Could you check a few things on this model? Use its own coordinates, in mm. Face numbers are marked on the shaded views. Give positions to 0.01 mm unless a question says otherwise; leave off trailing zeros. Order: outer loops, then holes, each group sorted by start corner. A loop starts at its lowest first (then second) coordinate and runs counter-clockwise, first axis right, second up.
(1) Imagine slicing it at A-A, the plane x = -0.5. Write out the boundary of the cut face in (y, z), then the cut area to 3 significant figures.
(2) Will these pins go through, and if not, where does the flat tip stop? pin 1 (3 mm diameter, centred on x = 11.5, z = -28.5, fed in from +Y); pin 2 (0.6 mm diameter, centred on y = 1.5, z = -25.5, fed in from -X); pin 3 (2 mm diameter, centred on y = 9, z = -24, fed in from -X).
(3) Imagine slicing it at C-C, the plane z = -13. Write out the boundary of the cut face in (x, y).
(4) If we mould it in two halves opening along Y, with no side actions, what happens to the marked faces 1, 2 and 3? For each: released by +Y, released by -Y, zero draft, split by the parting line, or undercut.
(5) Imagine slicing it at B-B, the plane y = 7. Write out the boundary of the cut face in (x, z).
(6) If I drill on probe 1 along X at (y, z) = (1, -34); probe 2 along Z at (x, y) = (15, 7.25); probe 3 along Y at (x, z) = (5.25, -31), over which ranges is the centre line in solid material (lowest first)?
(7) Imagine slicing it at D-D, the plane x = 2.5. Write out the boundary of the cut face in (y, z), then the cut area to 3 significant figures.
from build123d import *

# Parameters (mm, degrees)
SKETCH1_R           = 1.75
BOSS_EXTRUDE1_DEPTH = 2
SKETCH4_W           = 2
SKETCH4_H           = 36.35059407
BOSS_EXTRUDE3_DEPTH = 10
CUT_EXTRUDE1_DEPTH  = 10
FILLET1_R           = 3


with BuildPart() as part:
    # Sketch1 → Boss-Extrude1 (new body)
    with BuildSketch(Plane(origin=(0, 0, 0), x_dir=(1, 0, 0), z_dir=(0, 1, 0))):
        Polygon((5.603006234, 2.519255437), (16.866529546, 2.519255437), (16.866529546, 38.869849507), (4.37040298, 38.869849507), (-1.929271174, 38.869849507), (-1.929271174, 30.775756588), (6.866529546, 30.775756588), (6.866529546, 19.460556696), (-1.929271174, 19.460556696), (-1.929271174, 2.519255437), align=None)
        with Locations(Location((2.868105939, 34.070567936, 0), (0, 0, 270))):
            Circle(SKETCH1_R, mode=Mode.SUBTRACT)
        with Locations(Location((2.854801247, 6.270571119, 0), (0, 0, 270))):
            Circle(SKETCH1_R, mode=Mode.SUBTRACT)
    extrude(amount=BOSS_EXTRUDE1_DEPTH)

    # Sketch4 → Boss-Extrude3 (add)
    with BuildSketch(Plane(origin=(0, 2, 0), x_dir=(1, 0, 0), z_dir=(0, 1, 0))):
        with Locations((15.866529546, 20.694552472)):
            Rectangle(SKETCH4_W, SKETCH4_H)
    extrude(amount=BOSS_EXTRUDE3_DEPTH)

    # Sketch5 → Cut-Extrude1 (cut)
    with BuildSketch(Plane.ZY.offset(-14.866529546)):
        with BuildLine():
            Line((-5.270571119, 5.25), (-7.270571119, 5.25))
            ThreePointArc((-7.270571119, 5.25), (-9.020571119, 7), (-7.270571119, 8.75))
            Line((-7.270571119, 8.75), (-5.270571119, 8.75))
            ThreePointArc((-5.270571119, 8.75), (-3.520571119, 7), (-5.270571119, 5.25))
        make_face()
        with BuildLine():
            Line((-33.822803047, 5.25), (-35.822803047, 5.25))
            ThreePointArc((-35.822803047, 5.25), (-37.572803047, 7), (-35.822803047, 8.75))
            Line((-35.822803047, 8.75), (-33.822803047, 8.75))
            ThreePointArc((-33.822803047, 8.75), (-32.072803047, 7), (-33.822803047, 5.25))
        make_face()
    extrude(amount=-CUT_EXTRUDE1_DEPTH, mode=Mode.SUBTRACT)

    # Fillet1
    fillet1_edges = [part.edges().sort_by_distance(p)[0] for p in [
        (14.866529546, 2, -20.694552472),
    ]]
    fillet(fillet1_edges, radius=FILLET1_R)


solid = part.part
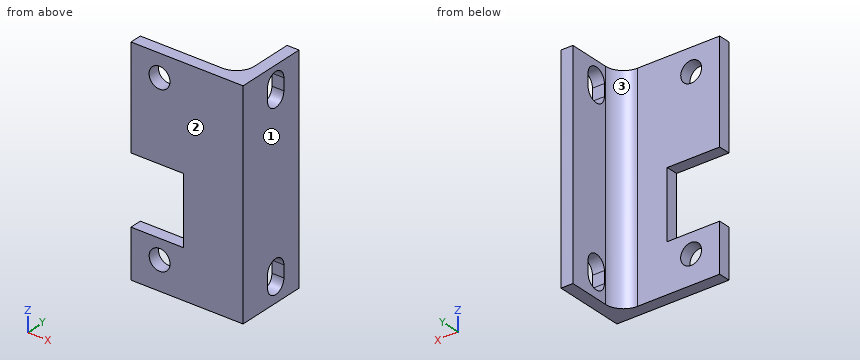
Answer block:
1. outline: (0, -38.87) - (2, -38.87) - (2, -30.78) - (0, -30.78) - close; (0, -19.46) - (2, -19.46) - (2, -2.52) - (0, -2.52) - close
1. area: 50.1 mm2
2. pin 1: stops at y = 2.22
2. pin 2: stops at x = 6.87
2. pin 3: stops at x = 14.87
3. outline: (-1.93, 0) - (16.87, 0) - (16.87, 12) - (14.87, 12) - (14.87, 5) arc R3 cw to (11.87, 2) - (-1.93, 2) - close
4. face 1: zero draft
4. face 2: released by -Y
4. face 3: released by +Y
5. outline: (14.87, -38.87) - (16.87, -38.87) - (16.87, -37.57) - (14.87, -37.57) - close; (14.87, -32.07) - (16.87, -32.07) - (16.87, -9.02) - (14.87, -9.02) - close; (14.87, -3.52) - (16.87, -3.52) - (16.87, -2.52) - (14.87, -2.52) - close
6. probe 1: x = -1.93 to 1.12, 4.62 to 16.87
6. probe 2: z = -38.87 to -37.55, -32.09 to -9, -3.54 to -2.52
6. probe 3: y = 0 to 2
7. outline: (0, -38.87) - (2, -38.87) - (2, -35.78) - (0, -35.78) - close; (0, -32.36) - (2, -32.36) - (2, -30.78) - (0, -30.78) - close; (0, -19.46) - (2, -19.46) - (2, -7.98) - (0, -7.98) - close; (0, -4.56) - (2, -4.56) - (2, -2.52) - (0, -2.52) - close
7. area: 36.4 mm2
